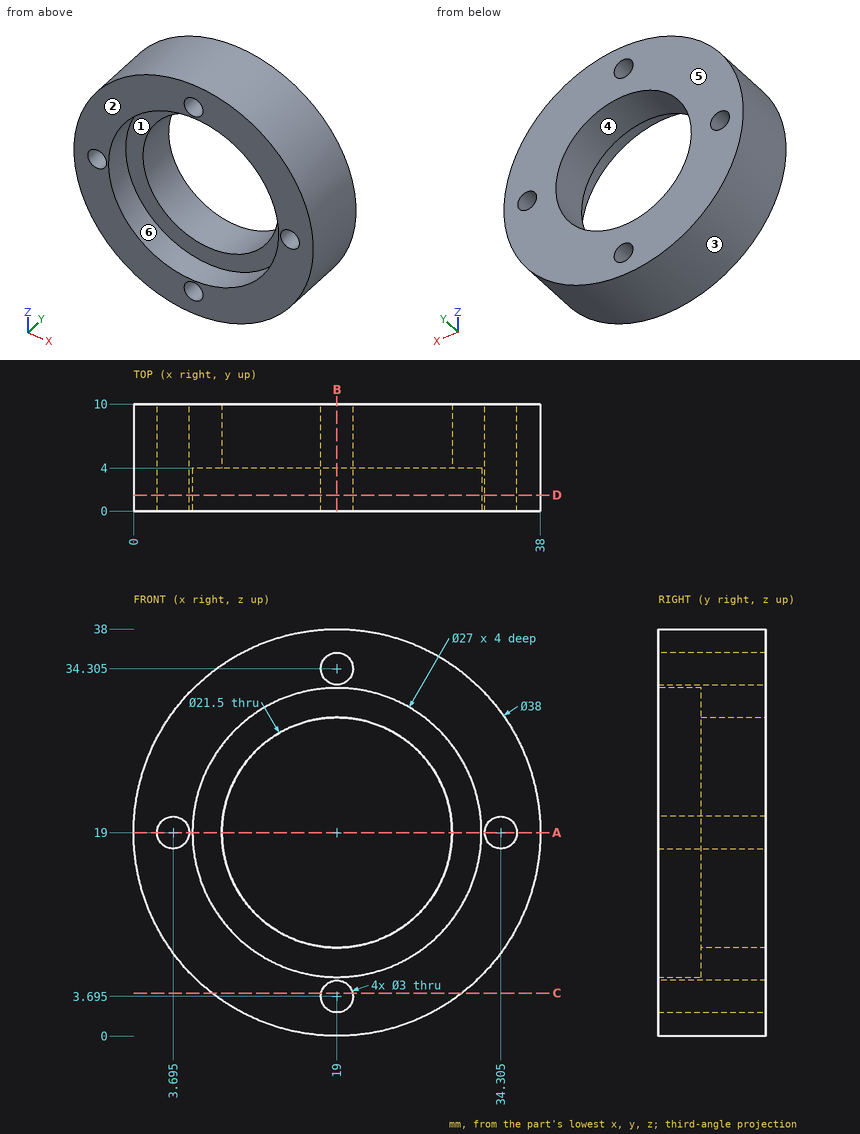
Job drawing, mm, ordinate dimensions from the low corner. One solid piece. A direction names the side the tool comes from. Coordinates: 2 decimals unless noted, no trailing zeros. Write each loop counter-clockwise with the first axis right and the second up, starting at its lowest first coordinate (ties: lowest second). Pieces come first, ordered by that corner, then holes. Notation, with made-up numbers: M -32.75,71 L -18.75,71 A9 ccw -18.75,79 Z; hole C 30.5,14 d11. An arc over 180 degrees is marked long. Answer as a JSON object with one key per item and string values. Group by question number.
1) Pin check, flat tips, straight feed: pin 1 Ø1 at (y, z) = (7.5, 7.5) entering from -X; pin 2 Ø3 at (y, z) = (7, 33) entering from -X; pin 3 Ø1 at (x, y) = (31.5, 1) entering from +Z. Stop position of each tip, or through.
2) Saw through at C-C (z = 4). Write the cut outline in (x, y), plus the area to 3 significant figures.
3) Wall check: line 1 (X direction, y = 3.25, z = 19) (3 decimals); line 2 (X direction, y = 5.75, z = 19) (3 decimals); line 3 (Z direction, x = 20, y = 8.5). Give the ranges that are in metal, low to high. Write a range as from..to.
4) Saw through at A-A (z = 19). Write the cut outline in (x, y) (3 decimals).
5) Mould opens along X. For the marked faces 1, 2, 3 and 4 say: +X half, -X half, draft (parallel to the pull), parting line (faces both ways), or undercut.
6) Saw through at B-B (x = 19). Write the cut outline in (y, z) (3 decimals).
7) Tool access for the marked faces 5 and 6: list every direction of +Z, -Z, +X, -X, +Y, -Y with a clear straight run to the whole face (end or side of a thin tool).
8) Saw through at D-D (y = 1.5). Write the cut outline in (x, z) (3 decimals), plus the area to 3 significant figures.
Values follow:
{
 "1": {"pin 1": "stops at x = 3.51", "pin 2": "stops at x = 4.69", "pin 3": "stops at z = 33.73"},
 "2": {"outline": "M 7.34,0 L 17.53,0 L 17.53,10 L 7.34,10 Z; M 20.47,0 L 30.66,0 L 30.66,10 L 20.47,10 Z", "area": "204 mm2"},
 "3": {"line 1": "x = 0..2.195, 5.195..5.5, 32.5..32.805, 35.805..38", "line 2": "x = 0..2.195, 5.195..8.25, 29.75..32.805, 35.805..38", "line 3": "z = 0.03..2.58, 4.81..8.3, 29.7..33.19, 35.42..37.97"},
 "4": {"outline": "M 0,0 L 2.195,0 L 2.195,10 L 0,10 Z; M 5.195,0 L 5.5,0 L 5.5,4 L 8.25,4 L 8.25,10 L 5.195,10 Z; M 29.75,4 L 32.5,4 L 32.5,0 L 32.805,0 L 32.805,10 L 29.75,10 Z; M 35.805,0 L 38,0 L 38,10 L 35.805,10 Z"},
 "5": {"face 1": "undercut", "face 2": "draft", "face 3": "parting line", "face 4": "undercut"},
 "6": {"outline": "M 0,0 L 10,0 L 10,2.195 L 0,2.195 Z; M 0,5.195 L 10,5.195 L 10,8.25 L 4,8.25 L 4,5.5 L 0,5.5 Z; M 0,32.5 L 4,32.5 L 4,29.75 L 10,29.75 L 10,32.805 L 0,32.805 Z; M 0,35.805 L 10,35.805 L 10,38 L 0,38 Z"},
 "7": {"face 5": "+Z, -Z, +X, -X, +Y", "face 6": "-Y"},
 "8": {"outline": "C 19,19 d38; hole C 3.695,19 d3; hole C 19,19 d27; hole C 19,3.695 d3; hole C 19,34.305 d3; hole C 34.305,19 d3", "area": "533 mm2"}
}
